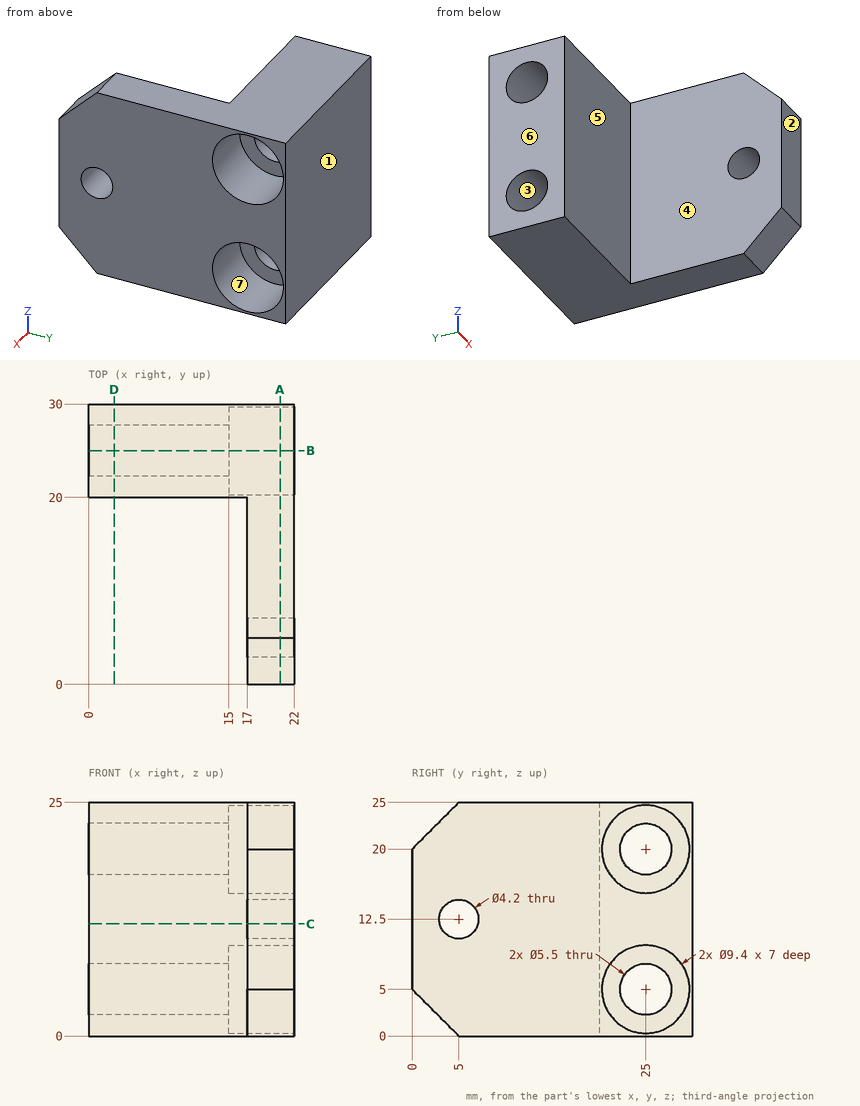
Answer from the drawing. Dimensions are ordinates in mm from the lowest x, y and z of the part. A direction names the side the tool comes from. Give positions to 0.01 mm unless a question says otherwise; leave off trailing zeros. Loops run counter-clockwise (first coordinate to the right, second up) from the corner with the lowest first, then second, coordinate; pieces in that order, holes last. Notation, with made-up numbers: (-10.75, 44.25) -> (47.25, 44.25) arc R19 ccw to (47.25, 58.25) -> close; hole circle Ø3 at (-19.5, 7). An arc over 180 degrees is marked (long way). One line per question, with ' | ' between items. Start each with the question number.
1) Section C-C, the plane z = 12 is taken. Determine the outline of the cut face in (x, y), then the cut area to 3 significant figures.
2) Straight lines are drawn through the part: L1, parallel to Y at x = 19.25, z = 20; L2, parallel to Y at x = 7, z = 20; L3, parallel to Z at x = 2.75, y = 25.75. For each, find the intervals that lie inside material, in ascending order.
3) Section D-D, the plane x = 2.75 is taken. Determine the outline of the cut face in (y, z).
4) Section B-B, the plane y = 25 is taken. Determine the outline of the cut face in (x, z), then the cut area to 3 significant figures.
5) Section A-A, the plane x = 20.5 is taken. Determine the outline of the cut face in (y, z).
6) Determine the mould class of the marked faces 1, 2, 3 and 4 for opening direction Y: +Y half, -Y half, draft (parallel to the pull), parting line (faces both ways), or undercut.
7) Each of these flat-tipped pins is pushed along its axis until it touches: pin 1 (12 mm diameter, centred on x = 10, y = 13, fed in from -Z); pin 2 (7 mm diameter, centred on y = 25, z = 5, fed in from +X); pin 3 (1 mm diameter, centred on y = 3.5, z = 10, fed in from -X). Where does it stop, or does it pass through?
8) For the marked faces 5, 6 and 7, determine the directions among +Z, -Z, +X, -X, +Y, -Y from which every point of the face is accessible in a straight line to the end or side of a thin tool.
Resolved:
1) outline: (0, 20) -> (17, 20) -> (17, 7.04) -> (22, 7.04) -> (22, 30) -> (0, 30) -> close; (17, 0) -> (22, 0) -> (22, 2.96) -> (17, 2.96) -> close | area: 300 mm2
2) L1: 0 to 20.3, 29.7 to 30 | L2: 20 to 22.25, 27.75 to 30 | L3: 0 to 2.35, 7.65 to 17.35, 22.65 to 25
3) outline: (20, 0) -> (30, 0) -> (30, 25) -> (20, 25) -> close; hole circle Ø5.5 at (25, 5); hole circle Ø5.5 at (25, 20)
4) outline: (0, 0) -> (22, 0) -> (22, 0.3) -> (15, 0.3) -> (15, 2.25) -> (0, 2.25) -> close; (0, 7.75) -> (15, 7.75) -> (15, 9.7) -> (22, 9.7) -> (22, 15.3) -> (15, 15.3) -> (15, 17.25) -> (0, 17.25) -> close; (0, 22.75) -> (15, 22.75) -> (15, 24.7) -> (22, 24.7) -> (22, 25) -> (0, 25) -> close | area: 253 mm2
5) outline: (0, 5) -> (5, 0) -> (30, 0) -> (30, 25) -> (5, 25) -> (0, 20) -> close; hole circle Ø4.2 at (5, 12.5); hole circle Ø9.4 at (25, 5); hole circle Ø9.4 at (25, 20)
6) face 1: +Y half | face 2: -Y half | face 3: undercut | face 4: draft
7) pin 1: through | pin 2: x = 15 | pin 3: x = 17
8) face 5: +Z, -Z, -X, -Y | face 6: +Z, -Z, -X, +Y, -Y | face 7: +X
